Build history of the part. All positions in model axes, mm. A direction names the side the tool comes from. Round coordinates to 2 decimals unless told otherwise and drop trailing zeros. Write each loop counter-clockwise with the first axis right and the second up, starting at its lowest first coordinate (ties: lowest second). Pieces come first, ordered by that corner, then holes. Notation, with made-up numbers: M -31.75,-35 L 22.25,-35 A15 cw 22.25,-29 Z; hole C 43.5,34 d2. An arc over 180 degrees is marked long. Use a Markdown table: item, result.
from build123d import *

# Parameters (mm, degrees)
F0_W     = 150
F0_H     = 144
F0_R     = 0.5
F1_DEPTH = 18
F2_R     = 0.5
F3_DEPTH = 1
F4_R     = 0.5
F5_DEPTH = 1
F6_W     = 18
F6_H     = 30
F7_DEPTH = 50
F8_W     = 18
F8_H     = 30
F9_DEPTH = 50


with BuildPart() as f1:
    # F0 (on Front) → F1 (new body)
    with BuildSketch(Plane.XZ):
        with Locations((75, 72)):
            Rectangle(F0_W, F0_H)
        with Locations((75, 17)):
            Circle(F0_R, mode=Mode.SUBTRACT)
        with Locations((75, 127)):
            Circle(F0_R, mode=Mode.SUBTRACT)
    extrude(amount=F1_DEPTH)

    # F2 (on face) → F3 (cut)
    with BuildSketch(Plane(origin=(0, 0, 0), x_dir=(1, 0, 0), z_dir=(0, 0, -1))):
        with Locations((75, 9)):
            Circle(F2_R)
    extrude(amount=-F3_DEPTH, mode=Mode.SUBTRACT)

    # F4 (on face) → F5 (cut)
    with BuildSketch(Plane.XY.offset(144)):
        with Locations((75, -9)):
            Circle(F4_R)
    extrude(amount=-F5_DEPTH, mode=Mode.SUBTRACT)

    # F6 (on face) → F7 (join)
    with BuildSketch(Plane(origin=(0, 0, 0), x_dir=(0, -1, 0), z_dir=(-1, 0, 0))):
        with Locations((9, 129)):
            Rectangle(F6_W, F6_H)
        with Locations((9, 15)):
            Rectangle(F6_W, F6_H)
    extrude(amount=F7_DEPTH)

    # F8 (on face) → F9 (join)
    with BuildSketch(Plane.YZ.offset(150)):
        with Locations((-9, 15)):
            Rectangle(F8_W, F8_H)
        with Locations((-9, 129)):
            Rectangle(F8_W, F8_H)
    extrude(amount=F9_DEPTH)


solid = f1.part
Q1. Cut at B-B on y = -2.75. Give the cut face in (x, z).
Response values:
| item | result |
|---|---|
| outline | M -50,0 L 200,0 L 200,30 L 150,30 L 150,114 L 200,114 L 200,144 L -50,144 L -50,114 L 0,114 L 0,30 L -50,30 Z; hole C 75,17 d1; hole C 75,127 d1 |
Q2. Cut at A-A on x = 168.5. Give the cut face in (y, z), and give its area (3 significant figures).
Response values:
| item | result |
|---|---|
| outline | M -18,0 L 0,0 L 0,30 L -18,30 Z; M -18,114 L 0,114 L 0,144 L -18,144 Z |
| area | 1,080 mm2 |
Q3. Drop flat-ended pins along their axis: P1, Ø0.8, axis at x = 75, y = -9, coming from the +Z side; P2, Ø5, axis at y = -7, z = 84, coming from the -X side; P3, Ø1.5, axis at y = -12, z = 42, coming from the +X side. Give the stop position or say it passes through.
Response values:
| item | result |
|---|---|
| P1 | stops at z = 143 |
| P2 | stops at x = 0 |
| P3 | stops at x = 150 |
Q4. Two-plate mould, pull along Z, no slides. Class faces 4 (the flat face through (73, -9, 0)), 5 (the flat face through (-50, -9, 129)), 6 (the flat face through (175, -9, 30)), 7 (the flat face through (77, -9, 144)): +Z half, -Z half, draft (parallel to the pull), parting line (faces both ways), or undercut.
Response values:
| item | result |
|---|---|
| face 4 | -Z half |
| face 5 | draft |
| face 6 | undercut |
| face 7 | +Z half |
Q5. Drill centre lines: L1, parallel to Z at x = 75, y = -11.5; L2, parallel to Y at x = 75, z = 143.5; L3, parallel to X at y = -6, z = 127. Where is each one in solid material? Low to high.
Response values:
| item | result |
|---|---|
| L1 | z = 0 to 16.5, 17.5 to 126.5, 127.5 to 144 |
| L2 | y = -18 to -9.5, -8.5 to 0 |
| L3 | x = -50 to 74.5, 75.5 to 200 |
Q6. Cut at C-C on z = 64. Give the cut face in (x, y).
Response values:
| item | result |
|---|---|
| outline | M 0,-18 L 150,-18 L 150,0 L 0,0 Z |
Q7. Which spindle directions (+Z, -Z, +X, -X, +Y, -Y) get a long thin tool onto all of the face, cutting with end or side? Do faces 1 (the flat face through (150, -9, 71)), 2 (the flat face through (-25, -9, 114)), 3 (the flat face through (-50, -9, 15)). Say none if no direction does.
Response values:
| item | result |
|---|---|
| face 1 | +X, +Y, -Y |
| face 2 | -X, +Y, -Y |
| face 3 | +Z, -Z, -X, +Y, -Y |
